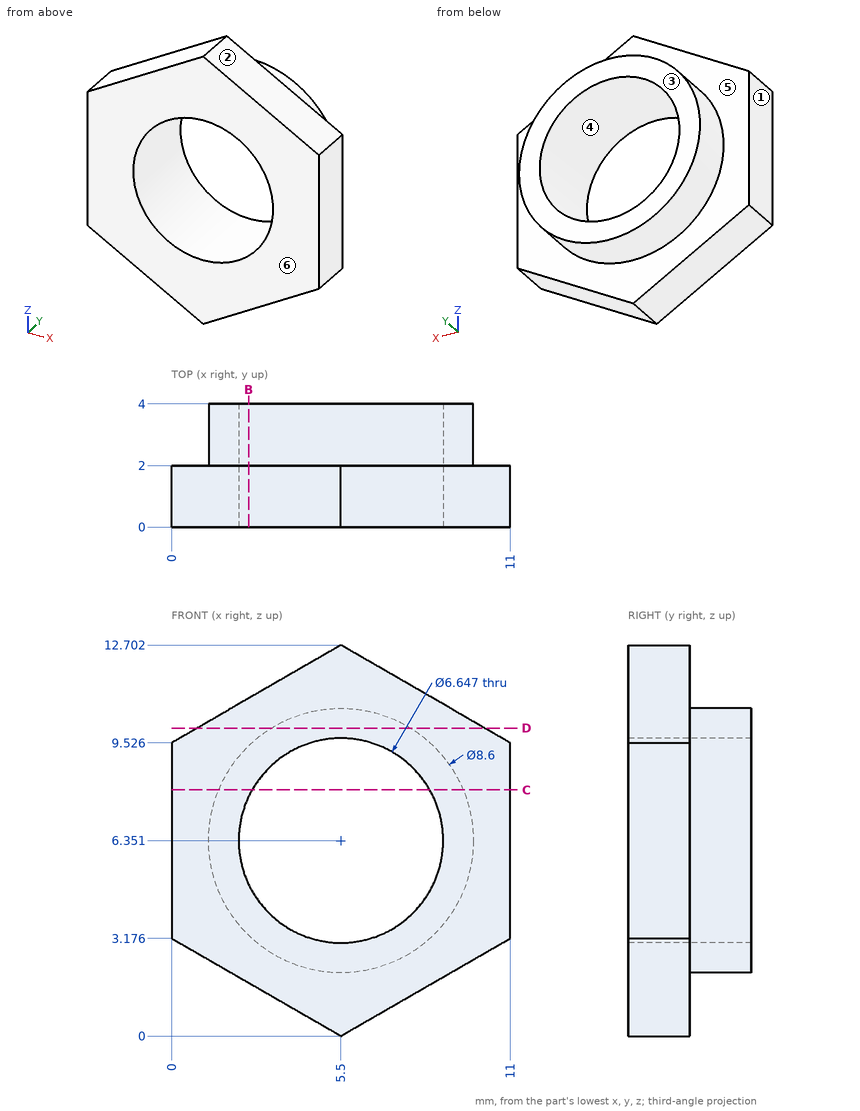
Design review of the part shown in the three views and the two pictorial views. Dimensions are in mm from the part's minimum x, y and z. A direction names the side the tool comes from. Round coordinates to 2 decimals unless told otherwise and drop trailing zeros. Write each loop counter-clockwise with the first axis right and the second up, starting at its lowest first coordinate (ties: lowest second). Pieces come first, ordered by that corner, then holes. Notation, with made-up numbers: (27.25, 89) - (37.25, 89) arc R16 cw to (37.25, 104) - close; hole circle Ø8 at (5.25, 5.25). An arc over 180 degrees is marked (long way). Return JSON: item names as keys, results as strings. Group by question number.
Item 1: We need section D-D on z = 10. Write out the cut boundary in (x, y) (1 decimal).
Item 2: Machinability: for the marked faces 5 and 6, which of the approach directions +Z, -Z, +X, -X, +Y, -Y give a long, thin tool a straight path to every point of the face, cutting with its end or side? Answer none if there is none.
Item 3: Insertion check: P1, Ø2, axis at y = 3.5, z = 2, coming from the -X side (1 decimal); P2, Ø2, axis at x = 7.5, y = 0.5, coming from the +Z side (1 decimal). Each pin has a flat end and moves straight along its axis. Give the tip position at first contact, or say it passes through.
Item 4: The part is to be moulded in two halves that separate along X. For the marked faces 1, 2, 3 and 4, say which applies: pulls with the +X half, pulls with the -X half, needs draft (parallel to the pull), parting line crosses it, or undercut.
Item 5: For probe 1 along X at (y, z) = (0.4, 6.25); probe 2 along X at (y, z) = (3.15, 7.5) (1 decimal); probe 3 along Y at (x, z) = (1.5, 9), list the stretches that pass through material, from the lowest coordinate up. Write a range as [from, to].
Item 6: We need section B-B on x = 2.5. Write out the cut boundary in (y, z).
Item 7: We need section C-C on z = 8. Write out the cut boundary in (x, y) (1 decimal).
Model answer:
{
 "1": {"outline": "(0.8, 0) - (10.2, 0) - (10.2, 2) - (7.8, 2) - (7.8, 4) - (3.2, 4) - (3.2, 2) - (0.8, 2) - close"},
 "2": {"face 5": "+Y", "face 6": "+Z, -Z, +X, -X, -Y"},
 "3": {"P1": "stops at x = 2.8", "P2": "stops at z = 12.1"},
 "4": {"face 1": "pulls with the -X half", "face 2": "pulls with the +X half", "face 3": "needs draft", "face 4": "undercut"},
 "5": {"probe 1": "x = [0, 2.18], [8.82, 11]", "probe 2": "x = [1.4, 2.4], [8.6, 9.6]", "probe 3": "y = [0, 2]"},
 "6": {"outline": "(0, 1.73) - (2, 1.73) - (2, 3.27) - (4, 3.27) - (4, 4.92) - (0, 4.92) - close; (0, 7.78) - (4, 7.78) - (4, 9.43) - (2, 9.43) - (2, 10.97) - (0, 10.97) - close"},
 "7": {"outline": "(0, 0) - (2.6, 0) - (2.6, 4) - (1.5, 4) - (1.5, 2) - (0, 2) - close; (8.4, 0) - (11, 0) - (11, 2) - (9.5, 2) - (9.5, 4) - (8.4, 4) - close"}
}
